Work out the finished part from the listing and answer in its coordinate system (mm). Round coordinates to 2 decimals unless told otherwise and drop trailing zeros. Write each loop counter-clockwise with the first axis right and the second up, starting at its lowest first coordinate (ties: lowest second). Pieces come first, ordered by that corner, then holes. Notation, with made-up numbers: (-12, 59.25) -> (45, 59.25) arc R25 ccw to (45, 97.25) -> close; hole circle Ø1 at (74.25, -22). An arc over 180 degrees is marked (long way). One line per item, written item: value.
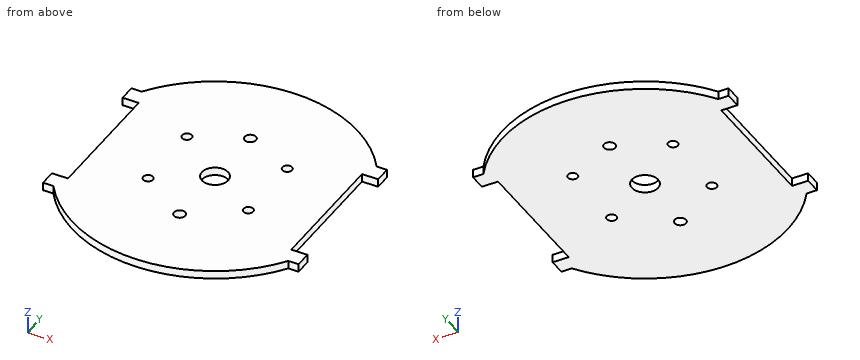
```python
from build123d import *

# Parameters (mm, degrees)
CROQUIS1_R              = 4.05
CROQUIS1_R_2            = 1.75
SALIENTE_EXTRUIR1_DEPTH = 2.5
CROQUIS2_R              = 1.5
CORTAR_EXTRUIR1_DEPTH   = 4


with BuildPart() as part:
    # Croquis1 → Saliente-Extruir1 (new body)
    with BuildSketch(Plane.XY):
        with BuildLine():
            Line((-39.500346279, 20), (-34.500346279, 20))
            Line((-34.500346279, 20), (-34.500346279, -20))
            Line((-34.500346279, -20), (-39.500346279, -20))
            Line((-39.500346279, -20), (-39.500346279, -25))
            Line((-39.500346279, -25), (-36.317049715, -25))
            ThreePointArc((-36.317049715, -25), (0, -44.09), (36.317049715, -25))
            Line((36.317049715, -25), (39.500346279, -25))
            Line((39.500346279, -25), (39.500346279, -20))
            Line((39.500346279, -20), (34.500346279, -20))
            Line((34.500346279, -20), (34.500346279, 20))
            Line((34.500346279, 20), (39.500346279, 20))
            Line((39.500346279, 20), (39.500346279, 25))
            Line((39.500346279, 25), (36.317049715, 25))
            ThreePointArc((36.317049715, 25), (0, 44.09), (-36.317049715, 25))
            Line((-36.317049715, 25), (-39.500346279, 25))
            Line((-39.500346279, 25), (-39.500346279, 20))
        make_face()
        Circle(CROQUIS1_R, mode=Mode.SUBTRACT)
        with Locations((0, 20)):
            Circle(CROQUIS1_R_2, mode=Mode.SUBTRACT)
        with Locations((0, -20)):
            Circle(CROQUIS1_R_2, mode=Mode.SUBTRACT)
    extrude(amount=SALIENTE_EXTRUIR1_DEPTH)

    # Croquis2 → Cortar-Extruir1 (cut)
    with BuildSketch(Plane(origin=(0, 0, 0), x_dir=(-1, 0, 0), z_dir=(0, 0, -1))):
        with Locations((15.5, -9.5)):
            Circle(CROQUIS2_R)
        with Locations((15.5, 12.5)):
            Circle(CROQUIS2_R)
        with Locations((-15.5, 12.5)):
            Circle(CROQUIS2_R)
        with Locations((-15.5, -9.5)):
            Circle(CROQUIS2_R)
    extrude(amount=-CORTAR_EXTRUIR1_DEPTH, mode=Mode.SUBTRACT)


solid = part.part
```
(1) Consider probe 1 along Y at (x, z) = (0, 0.75); probe 2 along Y at (x, z) = (-15.5, 1.6); probe 3 along Y at (x, z) = (1, 1.1). Determine where each line is inside the solid, lowest interval first.
Reported:
probe 1: y = -44.09 to -21.75, -18.25 to -4.05, 4.05 to 18.25, 21.75 to 44.09
probe 2: y = -41.28 to -11, -8 to 11, 14 to 41.28
probe 3: y = -44.08 to -21.44, -18.56 to -3.92, 3.92 to 18.56, 21.44 to 44.08
(2) Flat-ended cylindrical pins translate along their axes: pin 1 Ø1.5 at (x, z) = (30, 1) entering from +Y; pin 2 Ø0.8 at (x, z) = (-38, 1) entering from +Y; pin 3 Ø0.8 at (y, z) = (1, 1) entering from +X. Find the tip coordinate at first contact, or state that the pin passes through.
Reported:
pin 1: stops at y = 32.99
pin 2: stops at y = 25
pin 3: stops at x = 34.5
(3) Find section B-B on z = 2.05. Give the vertices of the cut face in (x, y).
Reported:
outline: (-39.5, -25) -> (-36.32, -25) arc R44.09 ccw to (36.32, -25) -> (39.5, -25) -> (39.5, -20) -> (34.5, -20) -> (34.5, 20) -> (39.5, 20) -> (39.5, 25) -> (36.32, 25) arc R44.09 ccw to (-36.32, 25) -> (-39.5, 25) -> (-39.5, 20) -> (-34.5, 20) -> (-34.5, -20) -> (-39.5, -20) -> close; hole circle Ø3 at (-15.5, -9.5); hole circle Ø3 at (-15.5, 12.5); hole circle Ø8.1 at (0, 0); hole circle Ø3.5 at (0, -20); hole circle Ø3.5 at (0, 20); hole circle Ø3 at (15.5, -9.5); hole circle Ø3 at (15.5, 12.5)
(4) Find section C-C on x = 0. Give the vertices of the cut face in (y, z), plus the area to 3 significant figures.
Reported:
outline: (-44.09, 0) -> (-21.75, 0) -> (-21.75, 2.5) -> (-44.09, 2.5) -> close; (-18.25, 0) -> (-4.05, 0) -> (-4.05, 2.5) -> (-18.25, 2.5) -> close; (4.05, 0) -> (18.25, 0) -> (18.25, 2.5) -> (4.05, 2.5) -> close; (21.75, 0) -> (44.09, 0) -> (44.09, 2.5) -> (21.75, 2.5) -> close
area: 183 mm2
(5) Find section A-A on y = 12.5. Give the vertices of the cut face in (x, z).
Reported:
outline: (-34.5, 0) -> (-17, 0) -> (-17, 2.5) -> (-34.5, 2.5) -> close; (-14, 0) -> (14, 0) -> (14, 2.5) -> (-14, 2.5) -> close; (17, 0) -> (34.5, 0) -> (34.5, 2.5) -> (17, 2.5) -> close
(6) Find section D-D on x = 15.5. Give the vertices of the cut face in (y, z).
Reported:
outline: (-41.28, 0) -> (-11, 0) -> (-11, 2.5) -> (-41.28, 2.5) -> close; (-8, 0) -> (11, 0) -> (11, 2.5) -> (-8, 2.5) -> close; (14, 0) -> (41.28, 0) -> (41.28, 2.5) -> (14, 2.5) -> close
